The listing builds one solid part. Answer for the finished solid, in the listing's coordinates (mm). Face numbers are marked on the shaded views. A direction names the side the tool comes from. Give positions to 0.01 mm unless a question says otherwise; leave off trailing zeros. Order: outer loops, then holes, each group sorted by start corner. A loop starts at its lowest first (then second) coordinate and runs counter-clockwise, first axis right, second up. Notation, with made-up numbers: (25.25, -28) - (81.25, -28) arc R30 ccw to (81.25, 3) - close; hole circle Ø8 at (-3, 43). An arc over 180 degrees is marked (long way). Write each question's results on one line, items separated by ' | '. Start each with the question number.
1. Flat-ended cylindrical pins translate along their axes: pin 1 (1.9 mm diameter, centred on x = 7.62, z = -3, fed in from +Y); pin 2 (3 mm diameter, centred on x = 0, z = 2, fed in from -Y); pin 3 (4.5 mm diameter, centred on y = 5, z = 0, fed in from +X); pin 4 (4 mm diameter, centred on y = 11.5, z = 8, fed in from -X). Find the tip coordinate at first contact, or state that the pin passes through.
2. Section A-A (y = 5) is taken. Give the vertices of the cut face in (x, z).
3. Which of the six approach directions +Z, -Z, +X, -X, +Y, -Y give full straight-line access (tool end or side, diameter ignored) to the marked faces 5 and 6?
4. Section C-C (x = 0) is taken. Give the vertices of the cut face in (y, z).
5. Section D-D (y = 21.75) is taken. Give the vertices of the cut face in (x, z), and give its area (3 significant figures).
6. Determine the mould class of the marked faces 1, 2, 3 and 4 for opening direction X: released by +X, released by -X, zero draft, split by the parting line, or undercut.
7. Find the intervals of material crossed by L1, parallel to X at y = 22, z = -3; L2, parallel to Z at x = 0, y = 6; L3, parallel to Z at x = -4, y = 21.5, in increasing order.
8. Section B-B (z = 0) is taken. Give the vertices of the cut face in (x, y).
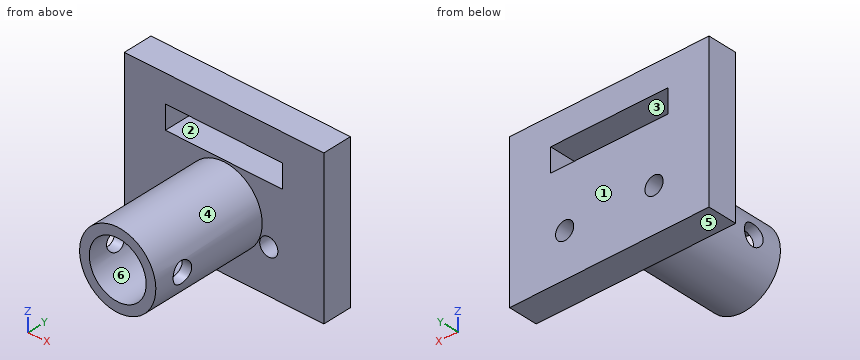
from build123d import *

# Parameters (mm, degrees)
SKETCH1_R               = 6.5
SKETCH1_R_2             = 4.85
BOSS_EXTRUDE1_DEPTH     = 25
SKETCH2_W               = 34
SKETCH2_H               = 26
BOSS_EXTRUDE2_DEPTH     = 5
CUT_EXTRUDE1_DEPTH      = 31.483602149
CUT_EXTRUDE1_DEPTH_BACK = 31.483602149
SKETCH3_R               = 1.55
SKETCH3_W               = 20
SKETCH3_H               = 4
CUT_EXTRUDE2_DEPTH      = 45.958314025
CUT_EXTRUDE2_DEPTH_BACK = 45.958314025
SKETCH4_R               = 1.75


with BuildPart() as part:
    # Sketch1 → Boss-Extrude1 (new body)
    with BuildSketch(Plane(origin=(0, 0, 0), x_dir=(1, 0, 0), z_dir=(0, 1, 0))):
        with Locations(Location((0, 0, 0), (0, 0, 270))):
            Circle(SKETCH1_R)
        with Locations(Location((0, 0, 0), (0, 0, 270))):
            Circle(SKETCH1_R_2, mode=Mode.SUBTRACT)
    extrude(amount=BOSS_EXTRUDE1_DEPTH)

    # Sketch2 → Boss-Extrude2 (add)
    with BuildSketch(Plane(origin=(0, 25, 0), x_dir=(1, 0, 0), z_dir=(0, 1, 0))):
        with Locations((0, -2.5)):
            Rectangle(SKETCH2_W, SKETCH2_H)
    extrude(amount=-BOSS_EXTRUDE2_DEPTH)

    # Sketch3 → Cut-Extrude1 (cut, two sides: drawn at the far end of the back side and taken through both)
    with BuildSketch(Plane(origin=(0, 20, 0), x_dir=(-1, 0, 0), z_dir=(0, -1, 0)).offset(-CUT_EXTRUDE1_DEPTH_BACK)):
        with Locations(Location((-7.62, 3, 0), (0, 0, 270))):
            Circle(SKETCH3_R)
        with Locations(Location((7.62, 3, 0), (0, 0, 270))):
            Circle(SKETCH3_R)
        with Locations((0, -8.8)):
            Rectangle(SKETCH3_W, SKETCH3_H)
    extrude(amount=CUT_EXTRUDE1_DEPTH + CUT_EXTRUDE1_DEPTH_BACK, mode=Mode.SUBTRACT)

    # Sketch4 → Cut-Extrude2 (cut, two sides: drawn at the far end of the back side and taken through both)
    with BuildSketch(Plane(origin=(17, 0, 0), x_dir=(0, 0, -1), z_dir=(1, 0, 0)).offset(-CUT_EXTRUDE2_DEPTH_BACK)):
        with Locations((0, 5)):
            Circle(SKETCH4_R)
    extrude(amount=CUT_EXTRUDE2_DEPTH + CUT_EXTRUDE2_DEPTH_BACK, mode=Mode.SUBTRACT)


solid = part.part
Reported:
1) pin 1: through | pin 2: y = 20 | pin 3: x = 6.5 | pin 4: x = -2.5
2) outline: (-6.26, -1.75) arc R6.5 ccw to (6.26, -1.75) - (4.52, -1.75) arc R4.85 cw to (-4.52, -1.75) - close; (-6.26, 1.75) - (-4.52, 1.75) arc R4.85 cw to (4.52, 1.75) - (6.26, 1.75) arc R6.5 ccw to start
3) face 5: -Z, +X, -X, +Y, -Y | face 6: -Y
4) outline: (0, -6.5) - (20, -6.5) - (20, -10.5) - (25, -10.5) - (25, 6.8) - (20, 6.8) - (20, 6.5) - (0, 6.5) - (0, 4.85) - (20, 4.85) - (20, -4.85) - (0, -4.85) - close; (20, 10.8) - (25, 10.8) - (25, 15.5) - (20, 15.5) - close
5) outline: (-17, -10.5) - (17, -10.5) - (17, 15.5) - (-17, 15.5) - close; hole (-10, 6.8) - (10, 6.8) - (10, 10.8) - (-10, 10.8) - close; hole circle Ø3.1 at (-7.62, -3); hole circle Ø3.1 at (7.62, -3) | area: 789 mm²
6) face 1: zero draft | face 2: undercut | face 3: undercut | face 4: split by the parting line
7) L1: -17 to -9.17, -6.07 to 6.07, 9.17 to 17 | L2: -6.5 to -4.85, 4.85 to 6.5 | L3: -10.5 to 6.8, 10.8 to 15.5
8) outline: (-17, 20) - (-6.5, 20) - (-6.5, 6.75) - (-4.85, 6.75) - (-4.85, 20) - (4.85, 20) - (4.85, 6.75) - (6.5, 6.75) - (6.5, 20) - (17, 20) - (17, 25) - (-17, 25) - close; (-6.5, 0) - (-4.85, 0) - (-4.85, 3.25) - (-6.5, 3.25) - close; (4.85, 0) - (6.5, 0) - (6.5, 3.25) - (4.85, 3.25) - close
